from build123d import *

# Parameters (mm, degrees)
SKETCH_110_R                     = 3.4
MEMBER_4080_2_0_4080_2_0_1_DEPTH = 1100
CUT_EXTRUDE_1_REACH              = 1104.297


with BuildPart() as part:
    # 草图110 → Member 4080-_2.0 _4080-_2.0_1 (new body)
    with BuildSketch(Plane(origin=(0, 0, 0), x_dir=(0, 0, -1), z_dir=(1, 0, 0))):
        with BuildLine():
            Line((-5.25, -3.977207794), (-5.25, 3.977207794))
            Line((-5.25, 3.977207794), (-11.522792206, 10.25))
            Line((-11.522792206, 10.25), (-18.2, 10.25))
            Line((-18.2, 10.25), (-18.2, 6.1))
            Line((-18.2, 6.1), (-17.3, 6.1))
            Line((-17.3, 6.1), (-17.3, 4.1))
            Line((-17.3, 4.1), (-18.8, 4.1))
            Line((-18.8, 4.1), (-18.8, 5.1))
            Line((-18.8, 5.1), (-20, 5.1))
            Line((-20, 5.1), (-20, 15.5))
            ThreePointArc((-20, 15.5), (-18.681980515, 18.681980515), (-15.5, 20))
            Line((-15.5, 20), (-5.1, 20))
            Line((-5.1, 20), (-5.1, 18.8))
            Line((-5.1, 18.8), (-4.1, 18.8))
            Line((-4.1, 18.8), (-4.1, 17.3))
            Line((-4.1, 17.3), (-6.1, 17.3))
            Line((-6.1, 17.3), (-6.1, 18.2))
            Line((-6.1, 18.2), (-10.25, 18.2))
            Line((-10.25, 18.2), (-10.25, 11.522792206))
            Line((-10.25, 11.522792206), (-3.977207794, 5.25))
            Line((-3.977207794, 5.25), (3.977207794, 5.25))
            Line((3.977207794, 5.25), (10.25, 11.522792206))
            Line((10.25, 11.522792206), (10.25, 18.2))
            Line((10.25, 18.2), (6.1, 18.2))
            Line((6.1, 18.2), (6.1, 17.3))
            Line((6.1, 17.3), (4.1, 17.3))
            Line((4.1, 17.3), (4.1, 18.8))
            Line((4.1, 18.8), (5.1, 18.8))
            Line((5.1, 18.8), (5.1, 20))
            Line((5.1, 20), (15.5, 20))
            Line((15.5, 20), (24.5, 20))
            Line((24.5, 20), (34.9, 20))
            Line((34.9, 20), (34.9, 18.8))
            Line((34.9, 18.8), (35.9, 18.8))
            Line((35.9, 18.8), (35.9, 17.3))
            Line((35.9, 17.3), (33.9, 17.3))
            Line((33.9, 17.3), (33.9, 18.2))
            Line((33.9, 18.2), (29.75, 18.2))
            Line((29.75, 18.2), (29.75, 11.522792206))
            Line((29.75, 11.522792206), (36.022792206, 5.25))
            Line((36.022792206, 5.25), (43.977207794, 5.25))
            Line((43.977207794, 5.25), (50.25, 11.522792206))
            Line((50.25, 11.522792206), (50.25, 18.2))
            Line((50.25, 18.2), (46.1, 18.2))
            Line((46.1, 18.2), (46.1, 17.3))
            Line((46.1, 17.3), (44.1, 17.3))
            Line((44.1, 17.3), (44.1, 18.8))
            Line((44.1, 18.8), (45.1, 18.8))
            Line((45.1, 18.8), (45.1, 20))
            Line((45.1, 20), (55.5, 20))
            ThreePointArc((55.5, 20), (58.681980515, 18.681980515), (60, 15.5))
            Line((60, 15.5), (60, 5.1))
            Line((60, 5.1), (58.8, 5.1))
            Line((58.8, 5.1), (58.8, 4.1))
            Line((58.8, 4.1), (57.3, 4.1))
            Line((57.3, 4.1), (57.3, 6.1))
            Line((57.3, 6.1), (58.2, 6.1))
            Line((58.2, 6.1), (58.2, 10.25))
            Line((58.2, 10.25), (51.522792206, 10.25))
            Line((51.522792206, 10.25), (45.25, 3.977207794))
            Line((45.25, 3.977207794), (45.25, -3.977207794))
            Line((45.25, -3.977207794), (51.522792206, -10.25))
            Line((51.522792206, -10.25), (58.2, -10.25))
            Line((58.2, -10.25), (58.2, -6.1))
            Line((58.2, -6.1), (57.3, -6.1))
            Line((57.3, -6.1), (57.3, -4.1))
            Line((57.3, -4.1), (58.8, -4.1))
            Line((58.8, -4.1), (58.8, -5.1))
            Line((58.8, -5.1), (60, -5.1))
            Line((60, -5.1), (60, -15.5))
            ThreePointArc((60, -15.5), (58.681980515, -18.681980515), (55.5, -20))
            Line((55.5, -20), (45.1, -20))
            Line((45.1, -20), (45.1, -18.8))
            Line((45.1, -18.8), (44.1, -18.8))
            Line((44.1, -18.8), (44.1, -17.3))
            Line((44.1, -17.3), (46.1, -17.3))
            Line((46.1, -17.3), (46.1, -18.2))
            Line((46.1, -18.2), (50.25, -18.2))
            Line((50.25, -18.2), (50.25, -11.522792206))
            Line((50.25, -11.522792206), (43.977207794, -5.25))
            Line((43.977207794, -5.25), (36.022792206, -5.25))
            Line((36.022792206, -5.25), (29.75, -11.522792206))
            Line((29.75, -11.522792206), (29.75, -18.2))
            Line((29.75, -18.2), (33.9, -18.2))
            Line((33.9, -18.2), (33.9, -17.3))
            Line((33.9, -17.3), (35.9, -17.3))
            Line((35.9, -17.3), (35.9, -18.8))
            Line((35.9, -18.8), (34.9, -18.8))
            Line((34.9, -18.8), (34.9, -20))
            Line((34.9, -20), (24.5, -20))
            Line((24.5, -20), (15.5, -20))
            Line((15.5, -20), (5.1, -20))
            Line((5.1, -20), (5.1, -18.8))
            Line((5.1, -18.8), (4.1, -18.8))
            Line((4.1, -18.8), (4.1, -17.3))
            Line((4.1, -17.3), (6.1, -17.3))
            Line((6.1, -17.3), (6.1, -18.2))
            Line((6.1, -18.2), (10.25, -18.2))
            Line((10.25, -18.2), (10.25, -11.522792206))
            Line((10.25, -11.522792206), (3.977207794, -5.25))
            Line((3.977207794, -5.25), (-3.977207794, -5.25))
            Line((-3.977207794, -5.25), (-10.25, -11.522792206))
            Line((-10.25, -11.522792206), (-10.25, -18.2))
            Line((-10.25, -18.2), (-6.1, -18.2))
            Line((-6.1, -18.2), (-6.1, -17.3))
            Line((-6.1, -17.3), (-4.1, -17.3))
            Line((-4.1, -17.3), (-4.1, -18.8))
            Line((-4.1, -18.8), (-5.1, -18.8))
            Line((-5.1, -18.8), (-5.1, -20))
            Line((-5.1, -20), (-15.5, -20))
            ThreePointArc((-15.5, -20), (-18.681980515, -18.681980515), (-20, -15.5))
            Line((-20, -15.5), (-20, -5.1))
            Line((-20, -5.1), (-18.8, -5.1))
            Line((-18.8, -5.1), (-18.8, -4.1))
            Line((-18.8, -4.1), (-17.3, -4.1))
            Line((-17.3, -4.1), (-17.3, -6.1))
            Line((-17.3, -6.1), (-18.2, -6.1))
            Line((-18.2, -6.1), (-18.2, -10.25))
            Line((-18.2, -10.25), (-11.522792206, -10.25))
            Line((-11.522792206, -10.25), (-5.25, -3.977207794))
        make_face()
        Circle(SKETCH_110_R, mode=Mode.SUBTRACT)
        with Locations((40, 0)):
            Circle(SKETCH_110_R, mode=Mode.SUBTRACT)
        with BuildLine():
            Line((-12.05, 12.05), (-18.2, 12.05))
            Line((-18.2, 12.05), (-18.2, 15.5))
            ThreePointArc((-18.2, 15.5), (-17.409188309, 17.409188309), (-15.5, 18.2))
            Line((-15.5, 18.2), (-12.05, 18.2))
            Line((-12.05, 18.2), (-12.05, 12.05))
        make_face(mode=Mode.SUBTRACT)
        Polygon((5.25, 3.977207794), (11.522792206, 10.25), (12.05, 10.777207794), (12.05, 12.05), (12.05, 18.2), (15.5, 18.2), (24.5, 18.2), (27.95, 18.2), (27.95, 12.05), (27.95, 10.777207794), (28.477207794, 10.25), (34.75, 3.977207794), (34.75, -3.977207794), (28.477207794, -10.25), (27.95, -10.777207794), (27.95, -12.05), (27.95, -18.2), (24.5, -18.2), (15.5, -18.2), (12.05, -18.2), (12.05, -12.05), (12.05, -10.777207794), (11.522792206, -10.25), (5.25, -3.977207794), align=None, mode=Mode.SUBTRACT)
        with BuildLine():
            Line((-12.05, -12.05), (-12.05, -18.2))
            Line((-12.05, -18.2), (-15.5, -18.2))
            ThreePointArc((-15.5, -18.2), (-17.409188309, -17.409188309), (-18.2, -15.5))
            Line((-18.2, -15.5), (-18.2, -12.05))
            Line((-18.2, -12.05), (-12.05, -12.05))
        make_face(mode=Mode.SUBTRACT)
        with BuildLine():
            Line((52.05, -12.05), (58.2, -12.05))
            Line((58.2, -12.05), (58.2, -15.5))
            ThreePointArc((58.2, -15.5), (57.409188309, -17.409188309), (55.5, -18.2))
            Line((55.5, -18.2), (52.05, -18.2))
            Line((52.05, -18.2), (52.05, -12.05))
        make_face(mode=Mode.SUBTRACT)
        with BuildLine():
            Line((52.05, 12.05), (52.05, 18.2))
            Line((52.05, 18.2), (55.5, 18.2))
            ThreePointArc((55.5, 18.2), (57.409188309, 17.409188309), (58.2, 15.5))
            Line((58.2, 15.5), (58.2, 12.05))
            Line((58.2, 12.05), (52.05, 12.05))
        make_face(mode=Mode.SUBTRACT)
    extrude(amount=MEMBER_4080_2_0_4080_2_0_1_DEPTH)

    # 草图13 → 切除-拉伸1 (cut, up to next)
    with BuildSketch(Plane(origin=(0, -18.2, 0), x_dir=(1, 0, 0), z_dir=(0, 1, 0)), mode=Mode.PRIVATE) as cut_extrude_1_sk1:
        with BuildLine():
            Line((1180, 11.75), (1100, 11.75))
            ThreePointArc((1100, 11.75), (1091.75, 20), (1100, 28.25))
            Line((1100, 28.25), (1180, 28.25))
            ThreePointArc((1180, 28.25), (1188.25, 20), (1180, 11.75))
        make_face()
    cut_extrude_1_tool1 = extrude(cut_extrude_1_sk1.sketch, amount=-CUT_EXTRUDE_1_REACH, mode=Mode.PRIVATE) & part.part
    add(cut_extrude_1_tool1.solids().sort_by_distance((1140, -18.2, -20))[0], mode=Mode.SUBTRACT)


solid = part.part
Geometry: final body of the model. Coordinates: model frame, mm. Round coordinates to 2 decimals unless told otherwise and drop trailing zeros.
Q1. Section A-A, the plane x = 423. Give the number of separate pieces and of enclosed holes in the cut face, and give its area (3 significant figures).
Result sheet:
separate pieces: 1
enclosed holes: 7
area: 747 mm2
Q2. Pin query (flat end, axial travel): pin 1 (0.5 mm diameter, centred on x = 386, z = 5, fed in from -Y); pin 2 (0.7 mm diameter, centred on x = 545.5, y = -17.5, fed in from -Z); pin 3 (10 mm diameter, centred on x = 309, z = -40, fed in from -Y); pin 4 (1 mm diameter, centred on y = 11, z = -13, fed in from -X). Return the tip coordinate at first contact, or that it passes through.
Result sheet:
pin 1: stops at y = -20
pin 2: stops at z = -59.69
pin 3: stops at y = -18.8
pin 4: passes through
Q3. Material intervals for probe 1 along Y at (x, z) = (840.5, -5); probe 2 along Y at (x, z) = (763.5, -55.5); probe 3 along Z at (x, y) = (153, -16.5), sorted ascending.
Result sheet:
probe 1: y = -18.8 to -17.3, -6.27 to 6.27, 17.3 to 18.8
probe 2: y = -20 to -18.2, -12.05 to -10.25, 10.25 to 12.05, 18.2 to 20
probe 3: z = -59.89 to -58.01, -52.05 to -50.25, -29.75 to -27.95, -12.05 to -10.25, 10.25 to 12.05, 18.01 to 19.89
